from build123d import *

# Parameters (mm, degrees)
PAD_DEPTH    = 8
SKETCH001_R  = 2.6
POCKET_DEPTH = 11.097152
FILLET_R     = 2
FILLET001_R  = 1


with BuildPart() as part:
    # Sketch → Pad (new body)
    with BuildSketch(Plane.XY):
        Polygon((-24.614359, 8), (24.614359, 8), (26.401924, 11.096152), (29, 9.596152), (26, 4.4), (28.944486, 2.7), (31.944486, 7.896152), (34.542563, 6.396152), (30.849742, 0), (-30.849742, 0), (-34.542563, 6.396152), (-31.944486, 7.896152), (-28.944486, 2.7), (-26, 4.4), (-29, 9.596152), (-26.401924, 11.096152), align=None)
    extrude(amount=PAD_DEPTH)

    # Sketch001 → Pocket (cut, through all)
    with BuildSketch(Plane.XZ):
        with Locations((0, 4)):
            Circle(SKETCH001_R)
    extrude(amount=-POCKET_DEPTH, mode=Mode.SUBTRACT)

    # Fillet
    fillet_edges = [part.edges().sort_by_distance(p)[0] for p in [
        (-30.849742, 0, 4),
        (-24.614359, 8, 4),
        (24.614359, 8, 4),
        (30.849742, 0, 4),
        (34.542563, 6.396152, 4),
        (26.401924, 11.096152, 4),
        (-26.401924, 11.096152, 4),
        (-34.542563, 6.396152, 4),
    ]]
    fillet(fillet_edges, radius=FILLET_R)

    # Fillet001
    fillet001_edges = [part.edges().sort_by_distance(p)[0] for p in [
        (0, 8, 0),
        (0, 0, 0),
        (0, 8, 8),
        (0, 0, 8),
    ]]
    fillet(fillet001_edges, radius=FILLET001_R)


solid = part.part
Design review of the part built by this model. Coordinates are the model's own, in mm. A direction names the side the tool comes from. Give positions to 0.01 mm unless a question says otherwise; leave off trailing zeros. Loops run counter-clockwise (first coordinate to the right, second up) from the corner with the lowest first, then second, coordinate; pieces in that order, holes last. Notation, with made-up numbers: M 12,-29 L 43,-29 A23 cw 43,-14 Z; hole C 20,38.25 d4. An arc over 180 degrees is marked long. Write item = value, one per line.
Q1. Insertion check: pin 1 (3 mm diameter, centred on y = 5, z = 6, fed in from -X); pin 2 (1 mm diameter, centred on y = 8, z = 5.5, fed in from +X); pin 3 (3 mm diameter, centred on y = 3, z = 2.5, fed in from +X); pin 4 (4 mm diameter, centred on x = -2.5, z = 2, fed in from +Y). Each pin has a flat end and moves straight along its axis. Give the tip position at first contact, or say it passes through.
Output values:
pin_1 = -33.81
pin_2 = 32.63
pin_3 = 33.45
pin_4 = 8
Q2. For faces 4 (the cylindrical face through (24.447, 8.261, 4.042)), 5 (the cylindrical face through (30.708, 0.275, 4.042)), 6 (the flat face through (-27.5, 7, 3.9)), list the 3-axis set-ups (+Z, -Z, +X, -X, +Y, -Y) from which the entire face can be reached by the end or side of a thin tool; tool diameter is ignored.
Output values:
face_4 = +Z, -Z, +Y
face_5 = +Z, -Z, +X, -Y
face_6 = +Z, -Z
Q3. We need section C-C (x = -20). Give the boundary of the cut face in (y, z), plus the area to 3 significant figures.
Output values:
outline = M 0,1 A1 ccw 1,0 L 7,0 A1 ccw 8,1 L 8,7 A1 ccw 7,8 L 1,8 A1 ccw 0,7 Z
area = 63.1 mm^2
Q4. We need section B-B (z = 3). Give the boundary of the cut face in (x, y).
Output values:
outline = M -33.54,4.66 L -31.43,1 A2 ccw -29.7,0 L -2.4,0 L -2.4,8 L -23.46,8 A2 cw -25.19,9 L -25.4,9.36 A2 ccw -28.13,10.1 L -29,9.6 L -26,4.4 L -28.94,2.7 L -31.94,7.9 L -32.81,7.4 A2 ccw Z; M 2.4,0 L 29.7,0 A2 ccw 31.43,1 L 33.54,4.66 A2 ccw 32.81,7.4 L 31.94,7.9 L 28.94,2.7 L 26,4.4 L 29,9.6 L 28.13,10.1 A2 ccw 25.4,9.36 L 25.19,9 A2 cw 23.46,8 L 2.4,8 Z
Q5. To check wall thickness, follow line 1 (Z direction, x = 0, y = 3.5); line 2 (X direction, y = 4.5, z = 3.5); line 3 (X direction, y = 5.75, z = 5.5). State the ranges of each line that lie inside material, in increasing order. Write a range as [from, to].
Output values:
line_1 = [0, 1.4], [6.6, 8]
line_2 = [-33.45, -29.98], [-26.06, -2.55], [2.55, 26.06], [29.98, 33.45]
line_3 = [-33.81, -30.71], [-26.78, -2.12], [2.12, 26.78], [30.71, 33.81]
Q6. Draft analysis for pull direction Z (two halves, no side actions). For faces 1 (the cylindrical face through (-0.338, 3.944, 6.578)), 2 (the flat face through (27.452, 3.562, 3.944)), 3 (the cylindrical face through (-28.42, 9.6, 0.3)), state which applies: +Z half, -Z half, draft (parallel to the pull), parting line (faces both ways), or undercut.
Output values:
face_1 = undercut
face_2 = draft
face_3 = -Z half
Q7. We need section A-A (x = 0). Give the boundary of the cut face in (y, z).
Output values:
outline = M 0,1 A1 ccw 1,0 L 7,0 A1 ccw 8,1 L 8,1.4 L 0,1.4 Z; M 0,6.6 L 8,6.6 L 8,7 A1 ccw 7,8 L 1,8 A1 ccw 0,7 Z
Q8. We need section D-D (z = 6). Give the boundary of the cut face in (x, y).
Output values:
outline = M -33.54,4.66 L -31.43,1 A2 ccw -29.7,0 L -1.66,0 L -1.66,8 L -23.46,8 A2 cw -25.19,9 L -25.4,9.36 A2 ccw -28.13,10.1 L -29,9.6 L -26,4.4 L -28.94,2.7 L -31.94,7.9 L -32.81,7.4 A2 ccw Z; M 1.66,0 L 29.7,0 A2 ccw 31.43,1 L 33.54,4.66 A2 ccw 32.81,7.4 L 31.94,7.9 L 28.94,2.7 L 26,4.4 L 29,9.6 L 28.13,10.1 A2 ccw 25.4,9.36 L 25.19,9 A2 cw 23.46,8 L 1.66,8 Z
